Can you work these out from the drawing? Everything is in mm from the part's minimum corner. A direction names the side the tool comes from. Coordinates: 2 decimals unless noted, no trailing zeros. Write each loop counter-clockwise with the first axis right and the second up, starting at its lowest first coordinate (ties: lowest second). Pieces come first, ordered by that corner, then holes. Notation, with made-up numbers: (40.25, 36.5) -> (50.25, 36.5) arc R14 cw to (50.25, 62.5) -> close; hole circle Ø2 at (37, 6). An arc over 180 degrees is marked (long way). Use a Markdown table: item, result. Add a question column.
Item 1: Imagine slicing it at D-D, the plane y = 1.5. Write out the boundary of the cut face in (x, z), and give its area (3 significant figures).
Item 2: If we mould it in two halves opening along X, with no side actions, what happens to the marked faces 5, 6 and 7? For each: pulls with the +X half, pulls with the -X half, needs draft (parallel to the pull), parting line crosses it, or undercut.
Item 3: Imagine slicing it at A-A, the plane x = 10. Write out the boundary of the cut face in (y, z).
Item 4: Imagine slicing it at B-B, the plane y = 15.75. Write out the boundary of the cut face in (x, z), and give its area (3 significant figures).
Item 5: If I drill on line 1 along X through (y, z) = (11.5, 2.5); line 2 along Y through (x, z) = (12.25, 0.75); line 3 along Y through (x, z) = (9.75, 0.7), over which ranges is the centre line in solid material (lowest first)? Write a range as from..to.
Item 6: On a 3-axis mill with a long thin cutter (end or side, diameter ignored), from which of +Z, -Z, +X, -X, +Y, -Y can I reach the whole of each face in a straight line? I mean the marked faces 1, 2, 3 and 4. Say none if no direction works.
Item 7: Will these pins go through, and if not, where does the flat tip stop? pin 1 Ø1 at (x, z) = (6, 0.5) entering from +Y; pin 2 Ø0.8 at (y, z) = (3, 4.5) entering from -X; pin 3 Ø2.5 at (x, y) = (9.5, 15) entering from +Z.
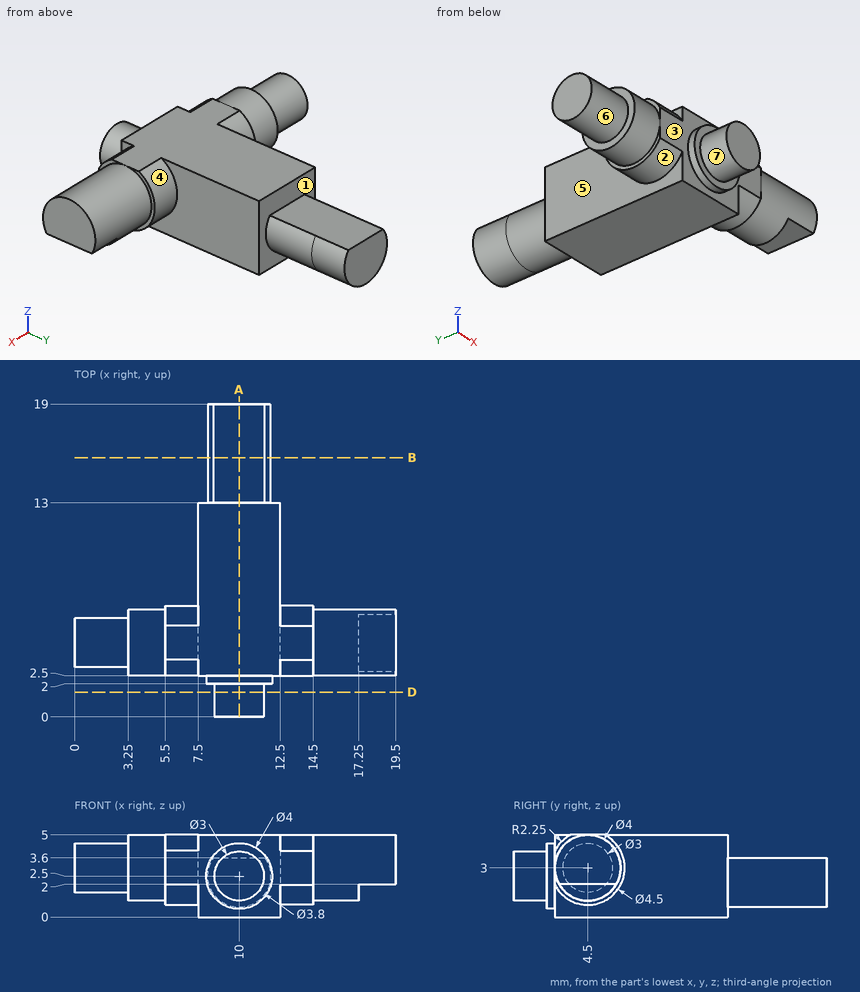
Ans:
| question | item | result |
|---|---|---|
| 1 | outline | circle Ø3 at (10, 2.5) |
| 1 | area | 7.07 mm^2 |
| 2 | face 5 | pulls with the -X half |
| 2 | face 6 | needs draft |
| 2 | face 7 | parting line crosses it |
| 3 | outline | (0, 1) -> (2, 1) -> (2, 0.5) -> (2.5, 0.5) -> (2.5, 0) -> (13, 0) -> (13, 0.6) -> (19, 0.6) -> (19, 3.6) -> (13, 3.6) -> (13, 5) -> (2.5, 5) -> (2.5, 4.5) -> (2, 4.5) -> (2, 4) -> (0, 4) -> close |
| 4 | outline | (8.45, 3.6) arc R1.9 ccw (long way) to (11.55, 3.6) -> close |
| 4 | area | 9.60 mm^2 |
| 5 | line 1 | x = 7.5..12.5 |
| 5 | line 2 | y = 2.5..13 |
| 5 | line 3 | y = 2..19 |
| 6 | face 1 | +Y |
| 6 | face 2 | -X |
| 6 | face 3 | -Y |
| 6 | face 4 | +X |
| 7 | pin 1 | stops at y = 5.53 |
| 7 | pin 2 | stops at x = 3.25 |
| 7 | pin 3 | stops at z = 3.6 |
